Here's how the part is built. I have some questions about the finished solid (model axes, mm). A direction names the side the tool comes from. Give positions to 0.01 mm unless a question says otherwise; leave off trailing zeros. Order: outer loops, then holes, each group sorted by start corner. A loop starts at its lowest first (then second) coordinate and runs counter-clockwise, first axis right, second up. Notation, with made-up numbers: M 2,48.5 L 15,48.5 A13 cw 15,71.5 Z; hole C -28.5,84 d4. An arc over 180 degrees is marked long. Use one line per item in the form item = value.
Autodesk Inventor part; units mm, degrees
ref_plane "YZ Plane" through (0, 0, 0) normal (1, 0, 0) x (0, 1, 0)
ref_plane "XZ Plane" through (0, 0, 0) normal (0, 1, 0) x (-1, 0, 0)
ref_plane "XY Plane" through (0, 0, 0) normal (0, 0, 1) x (1, 0, 0)
sketch "Sketch1" plane through (0, 0, 0) normal (0, 0, 1) x (1, 0, 0)
  circle A0 centre (0, 0) radius 3.4
  line L0 (0, 0) -> (20, 20) construction
  line L1 (0, 0) -> (28.2843, 0) construction
  line L2 (20, 20) -> (4.15, 20)
  line L3 (4.15, 20) -> (4.15, 15.5)
  line L4 (4.15, 15.5) -> (7.1, 15.5)
  line L5 (7.1, 15.5) -> (7.1, 18)
  line L6 (7.1, 18) -> (10.25, 18)
  line L7 (10.25, 18) -> (10.25, 14)
  line L8 (0, 0) -> (0, 26.1056) construction
  line L9 (10.25, 14) -> (2.3, 6.05)
  line L10 (2.3, 6.05) -> (0, 6.05)
  circle A1 centre (15, 15) radius 3
  line L11 (20, 20) -> (20, 4.15)
  line L12 (20, 4.15) -> (15.5, 4.15)
  line L13 (15.5, 4.15) -> (15.5, 7.1)
  line L14 (15.5, 7.1) -> (18, 7.1)
  line L15 (18, 7.1) -> (18, 10.25)
  line L16 (18, 10.25) -> (14, 10.25)
  line L17 (14, 10.25) -> (6.05, 2.3)
  line L18 (6.05, 2.3) -> (6.05, 0)
  line L19 (-2.3, 6.05) -> (0, 6.05)
  line L20 (-10.25, 14) -> (-2.3, 6.05)
  line L21 (-10.25, 18) -> (-10.25, 14)
  line L22 (-4.15, 15.5) -> (-7.1, 15.5)
  line L23 (-7.1, 15.5) -> (-7.1, 18)
  line L24 (-7.1, 18) -> (-10.25, 18)
  line L25 (-4.15, 20) -> (-4.15, 15.5)
  line L26 (-20, 20) -> (-4.15, 20)
  circle A2 centre (-15, 15) radius 3
  line L27 (-20, 20) -> (-20, 4.15)
  line L28 (-14, 10.25) -> (-6.05, 2.3)
  line L29 (-18, 7.1) -> (-18, 10.25)
  line L30 (-18, 10.25) -> (-14, 10.25)
  line L31 (-20, 4.15) -> (-15.5, 4.15)
  line L32 (-15.5, 4.15) -> (-15.5, 7.1)
  line L33 (-15.5, 7.1) -> (-18, 7.1)
  line L34 (-6.05, 2.3) -> (-6.05, 0)
  line L35 (-6.05, -2.3) -> (-6.05, 0)
  line L36 (-14, -10.25) -> (-6.05, -2.3)
  line L37 (-18, -10.25) -> (-14, -10.25)
  line L38 (-15.5, -4.15) -> (-15.5, -7.1)
  line L39 (-15.5, -7.1) -> (-18, -7.1)
  line L40 (-18, -7.1) -> (-18, -10.25)
  line L41 (-20, -4.15) -> (-15.5, -4.15)
  line L42 (-20, -20) -> (-20, -4.15)
  circle A3 centre (-15, -15) radius 3
  line L43 (-20, -20) -> (-4.15, -20)
  line L44 (-10.25, -14) -> (-2.3, -6.05)
  line L45 (-7.1, -18) -> (-10.25, -18)
  line L46 (-10.25, -18) -> (-10.25, -14)
  line L47 (-4.15, -20) -> (-4.15, -15.5)
  line L48 (-4.15, -15.5) -> (-7.1, -15.5)
  line L49 (-7.1, -15.5) -> (-7.1, -18)
  line L50 (-2.3, -6.05) -> (0, -6.05)
  line L51 (2.3, -6.05) -> (0, -6.05)
  line L52 (10.25, -14) -> (2.3, -6.05)
  line L53 (10.25, -18) -> (10.25, -14)
  line L54 (4.15, -15.5) -> (7.1, -15.5)
  line L55 (7.1, -15.5) -> (7.1, -18)
  line L56 (7.1, -18) -> (10.25, -18)
  line L57 (4.15, -20) -> (4.15, -15.5)
  line L58 (20, -20) -> (4.15, -20)
  circle A4 centre (15, -15) radius 3
  line L59 (20, -20) -> (20, -4.15)
  line L60 (14, -10.25) -> (6.05, -2.3)
  line L61 (18, -7.1) -> (18, -10.25)
  line L62 (18, -10.25) -> (14, -10.25)
  line L63 (20, -4.15) -> (15.5, -4.15)
  line L64 (15.5, -4.15) -> (15.5, -7.1)
  line L65 (15.5, -7.1) -> (18, -7.1)
  line L66 (6.05, -2.3) -> (6.05, 0)
  point P0 (0, 6.05)
  point P1 (-6.05, 0)
  point P2 (0, -6.05)
  dimension "d0" = 6.8
  dimension "d1" = 45
  dimension "d2" = 20
  dimension "d3" = 6
  dimension "d4" = 15
  dimension "d5" = 10.25
  dimension "d6" = 7.1
  dimension "d7" = 4.15
  dimension "d8" = 4.5
  dimension "d9" = 2
  dimension "d10" = 13.95
  dimension "d11" = 6
  dimension "d14" = 360
extrude "Extrusion1" add sketch "Sketch1" along normal blind 40
sketch "Sketch3" plane through (20, -20, 0) normal (1, 0, 0) x (0, 0, -1)
  line L0 (-14.5, 15.85) -> (-14.5, 0) construction
  line L1 (-20.5, 18.85) -> (-20.5, -3)
  line L2 (-8.5, 18.85) -> (-8.5, -3)
  line L3 (0, 15.85) -> (-40, 15.85)
  line L4 (0, 0) -> (-40, 0)
  line L5 (0, 0) -> (0, 15.85)
  line L6 (-20.5, 18.85) -> (-8.5, 18.85)
  line L7 (-20.5, -3) -> (-8.5, -3)
  point P0 (0, 20)
  dimension "d22" = 14.5
  dimension "d23" = 12
  dimension "d24" = 3
  dimension "d25" = 3
extrude "Extrusion3" cut sketch "Sketch3" against normal up to surface (13.95 mm away) contours L6 L2 L3 L1 | L3 L2 L4 L1 | L4 L2 L7 L1
properties part number "Aluminum_Profile_4040_40.10mm_left" material "Aluminum 6061-AHC"
Q1. I want a section at D-D on z = 12.5. State how many separate pieces and enclosed holes the cut face has, then the cut area to 3 significant figures.
Found:
separate_pieces = 2
enclosed_holes = 4
area = 580 mm²
Q2. I need wall thicknesses on L1, parallel to Y at x = -15, z = 12.5; L2, parallel to X at y = 6.5, z = 10; L3, parallel to Y at x = -17.5, z = 8.5. Which ranges of each line are inside material? Lowest first, please.
Found:
L1 = -20 to -18, -12 to -10.25, 10.25 to 12, 18 to 20
L2 = -20 to -15.5, -10.25 to -2.75, 2.75 to 10.25, 15.5 to 20
L3 = -20 to -16.66, -13.34 to -10.25, -7.1 to -4.15, 4.15 to 7.1, 10.25 to 13.34, 16.66 to 20
Q3. I'm going to push a flat-ended pin straight in: pin 1 Ø1.6 at (x, z) = (8.5, 11.5) entering from -Y. Where does the tip first touch, or does it pass through?
Found:
pin_1 = 3.95
Q4. I want a section at B-B on y = 0. Write out the boundary of the cut face in (x, z), then the cut area to 3 significant figures.
Found:
outline = M -6.05,0 L -3.4,0 L -3.4,40 L -6.05,40 Z; M 3.4,0 L 6.05,0 L 6.05,40 L 3.4,40 Z
area = 212 mm²
Q5. On a 3-axis mill with a long thin cutter (end or side, diameter ignored), from which of +Z, -Z, +X, -X, +Y, -Y can I reach the whole of each face in a straight line? I mean faces 4 (the face through (-6.05, 0, 20)), 5 (the face through (18, -9, 4)), 6 (the face through (18, -4.15, 4)). Say none if no direction works.
Found:
face_4 = +Z, -Z, -X
face_5 = +Z, -Z
face_6 = +Z, -Z, +X
Q6. Thinking about a two-plate mould opening in Y: for faces 1 (the face through (12, 20, 20)), 2 (the face through (-15.5, 6, 20)), 3 (the face through (0, 5, 40)), which applies, +Y half, -Y half, draft (parallel to the pull), parting line (faces both ways), or undercut?
Found:
face_1 = +Y half
face_2 = undercut
face_3 = draft
Q7. I want a section at A-A on x = -8.5. Write out the boundary of the cut face in (y, z).
Found:
outline = M -20,0 L -18,0 L -18,40 L -20,40 Z; M -12.25,0 L -4.75,0 L -4.75,40 L -12.25,40 Z; M 4.75,0 L 12.25,0 L 12.25,40 L 4.75,40 Z; M 18,0 L 20,0 L 20,40 L 18,40 Z
